from build123d import *

# Parameters (mm, degrees)
SKETCH1_W           = 84.5
SKETCH1_H           = 17.5
BOSS_EXTRUDE1_DEPTH = 1
FILLET1_R           = 3
SKETCH2_R           = 6
BOSS_EXTRUDE2_DEPTH = 13
SKETCH4_R           = 6
SKETCH4_R_2         = 4.7
CUT_EXTRUDE1_DEPTH  = 5


with BuildPart() as part:
    # Sketch1 → Boss-Extrude1 (new body)
    with BuildSketch(Plane.XY):
        with Locations((42.25, 8.75)):
            Rectangle(SKETCH1_W, SKETCH1_H)
        with BuildLine():
            Line((50.6, 13.1), (77.9, 13.1))
            ThreePointArc((77.9, 13.1), (81, 10), (77.9, 6.9))
            Line((77.9, 6.9), (50.6, 6.9))
            ThreePointArc((50.6, 6.9), (47.5, 10), (50.6, 13.1))
        make_face(mode=Mode.SUBTRACT)
        with BuildLine():
            Line((33.9, 13.1), (6.6, 13.1))
            ThreePointArc((6.6, 13.1), (3.5, 10), (6.6, 6.9))
            Line((6.6, 6.9), (33.9, 6.9))
            ThreePointArc((33.9, 6.9), (37, 10), (33.9, 13.1))
        make_face(mode=Mode.SUBTRACT)
    extrude(amount=BOSS_EXTRUDE1_DEPTH)

    # Fillet1
    fillet1_edges = [part.edges().sort_by_distance(p)[0] for p in [
        (0, 17.5, 0.5),
        (84.5, 17.5, 0.5),
        (84.5, 0, 0.5),
        (0, 0, 0.5),
    ]]
    fillet(fillet1_edges, radius=FILLET1_R)

    # Sketch2 → Boss-Extrude2 (add)
    with BuildSketch(Plane.XY.offset(1)):
        with Locations(Location((7.75, 10, 0), (0, 0, 31.108922511))):
            Circle(SKETCH2_R)
    boss_extrude2 = extrude(amount=BOSS_EXTRUDE2_DEPTH)

    # Sketch4 → Cut-Extrude1 (cut)
    with BuildSketch(Plane.XY.offset(1)):
        with Locations(Location((7.75, 10, 0), (0, 0, 180))):
            Circle(SKETCH4_R)
        with Locations(Location((7.75, 10, 0), (0, 0, 318.732572619))):
            Circle(SKETCH4_R_2, mode=Mode.SUBTRACT)
    cut_extrude1 = extrude(amount=CUT_EXTRUDE1_DEPTH, mode=Mode.SUBTRACT)

    # Mirror1: Boss-Extrude2, Cut-Extrude1 across plane
    add(boss_extrude2.mirror(Plane(origin=(42.25, 0, 0), x_dir=(0, 0, 1), z_dir=(1, 0, 0))))
    add(cut_extrude1.mirror(Plane(origin=(42.25, 0, 0), x_dir=(0, 0, 1), z_dir=(1, 0, 0))), mode=Mode.SUBTRACT)


solid = part.part
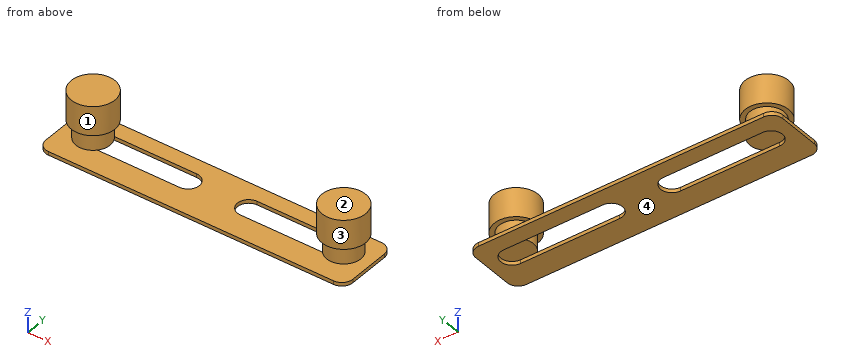
The model under review builds one solid part; all positions refer to its coordinate system, in mm. Face numbers are marked on the shaded views. A direction names the side the tool comes from. Give positions to 0.01 mm unless a question says otherwise; leave off trailing zeros. Order: outer loops, then holes, each group sorted by start corner. A loop starts at its lowest first (then second) coordinate and runs counter-clockwise, first axis right, second up. Notation, with made-up numbers: (60.25, 68) -> (70.25, 68) arc R24 ccw to (70.25, 88) -> close; hole circle Ø5 at (50.25, 78.5). An arc over 180 degrees is marked (long way). Write item = value, one per line. Start each with the question number.
(1) Take a section at B-B (x = 56). Write out the cut boundary in (y, z).
(2) Take a section at C-C (x = 7.75). Write out the cut boundary in (y, z).
(3) For L1, parallel to Z at x = 73, y = 14.25; L2, parallel to Z at x = 25.5, y = 1.25; L3, parallel to Z at x = 75, y = 12.75, list the stretches that pass through material, from the lowest coordinate up. Write a range as from..to.
(4) Take a section at D-D (z = 11.5). Write out the cut boundary in (x, y), plus the area to 3 significant figures.
(5) Tool access review of the marked faces 1 and 2: name each direction out of +Z, -Z, +X, -X, +Y, -Y from which nothing blocks a thin tool from reaching the whole face with its end or side.
(6) Draft analysis for pull direction X (two halves, no side actions). For the marked faces 3 and 4, state which applies: +X half, -X half, draft (parallel to the pull), parting line (faces both ways), or undercut.
(7) Take a section at A-A (y = 10). Write out the cut boundary in (x, z), plus the area to 4 significant figures.
(8) For pin 1 Ø8 at (x, z) = (71, 7) entering from +Y; pin 2 Ø1.5 at (y, z) = (6, 2) entering from -X; pin 3 Ø6 at (x, y) = (61, 10.5) entering from +Z, all flat-tipped, find the tip position at first contact; note any pin that passes through.
Returned:
q1.outline = (0, 0) -> (6.9, 0) -> (6.9, 1) -> (0, 1) -> close; (13.1, 0) -> (17.5, 0) -> (17.5, 1) -> (13.1, 1) -> close
q2.outline = (0, 0) -> (6.9, 0) -> (6.9, 1) -> (13.1, 1) -> (13.1, 0) -> (17.5, 0) -> (17.5, 1) -> (14.7, 1) -> (14.7, 6) -> (16, 6) -> (16, 14) -> (4, 14) -> (4, 6) -> (5.3, 6) -> (5.3, 1) -> (0, 1) -> close
q3.L1 = 0..1, 6..14
q3.L2 = 0..1
q3.L3 = 1..14
q4.outline = circle Ø12 at (7.75, 10); circle Ø12 at (76.75, 10)
q4.area = 226 mm²
q5.face_1 = +Z
q5.face_2 = +Z, +X, -X, +Y, -Y
q6.face_3 = undercut
q6.face_4 = draft
q7.outline = (0, 0) -> (3.5, 0) -> (3.5, 1) -> (12.45, 1) -> (12.45, 6) -> (13.75, 6) -> (13.75, 14) -> (1.75, 14) -> (1.75, 6) -> (3.05, 6) -> (3.05, 1) -> (0, 1) -> close; (37, 0) -> (47.5, 0) -> (47.5, 1) -> (37, 1) -> close; (70.75, 6) -> (72.05, 6) -> (72.05, 1) -> (81, 1) -> (81, 0) -> (84.5, 0) -> (84.5, 1) -> (81.45, 1) -> (81.45, 6) -> (82.75, 6) -> (82.75, 14) -> (70.75, 14) -> close
q7.area = 303.5 mm²
q8.pin_1 = 15.74
q8.pin_2 = 4.35
q8.pin_3 = 1
